Design review of the part shown in the three views and the two pictorial views. Dimensions are in mm from the part's minimum x, y and z. Coordinates: 2 decimals unless noted, no trailing zeros. Loops run counter-clockwise (first coordinate to the right, second up) from the corner with the lowest first, then second, coordinate; pieces in that order, holes last. Notation, with made-up numbers: (11.5, 31.25) - (15.5, 31.25) arc R21 ccw to (15.5, 47.25) - close; hole circle Ø6 at (16.5, -19.75). An arc over 180 degrees is marked (long way). One line per item, written item: value. Start each with the question number.
1. To check wall thickness, follow line 1 (Y direction, x = 25, z = 3.65); line 2 (Y direction, x = 15, z = 3.05); line 3 (Y direction, x = 2.25, z = 2.4). State the ranges of each line that lie inside material, in increasing order. Write a range as from..to.
2. Take a section at B-B, the plane z = 1.7. State the section outline as (x, y) points, and give its area (3 significant figures).
3. Insertion check: pin 1 (5 mm diameter, centred on x = 25, y = 112.5, fed in from +Z); pin 2 (1.5 mm diameter, centred on y = 123, z = 3.5, fed in from -X); pin 3 (2 mm diameter, centred on y = 26, z = 1.5, fed in from +X). Each pin has a flat end and moves straight along its axis. Give the tip position at first contact, or say it passes through.
4. Take a section at A-A, the plane x = 5. State the section outline as (y, z) points, and give its area (3 significant figures).
5. Take a section at C-C, the plane y = 12.5. State the section outline as (x, z) points.
6. Take a section at D-D, the plane x = 15. State the section outline as (y, z) points, and give its area (3 significant figures).
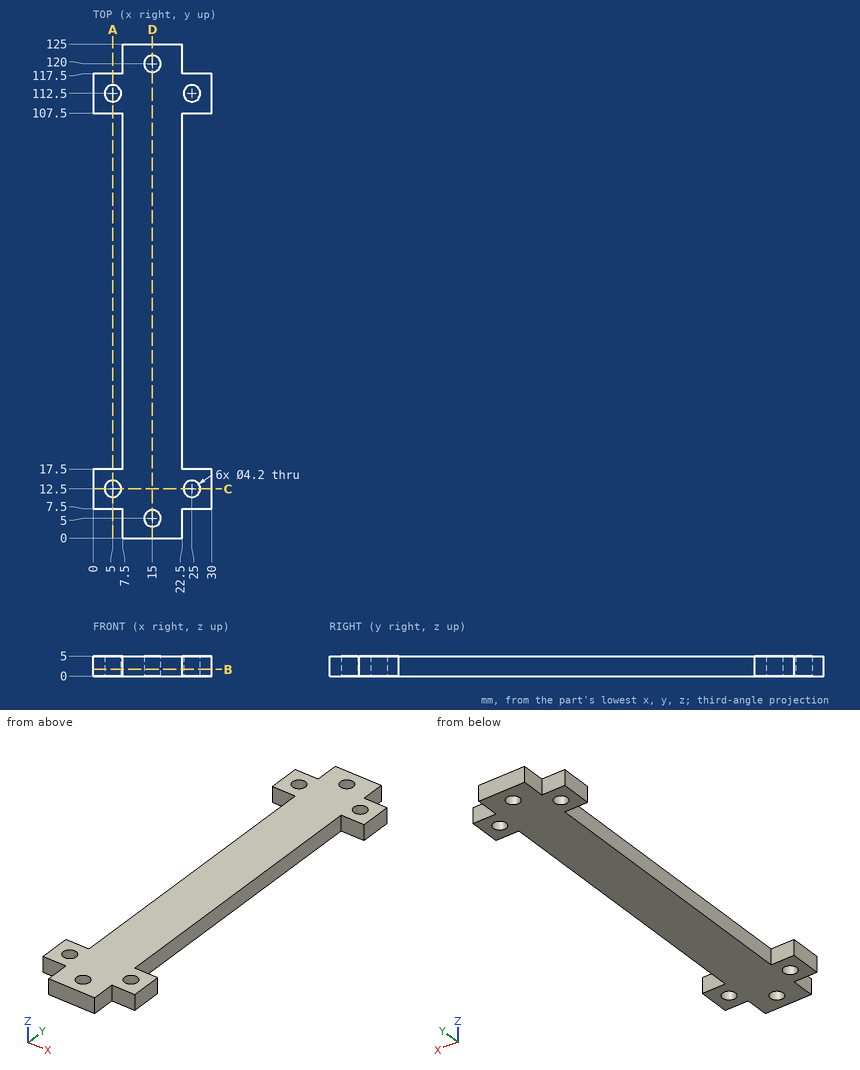
Solutions:
1. line 1: 7.5..10.4, 14.6..17.5, 107.5..110.4, 114.6..117.5
1. line 2: 0..2.9, 7.1..117.9, 122.1..125
1. line 3: 7.5..17.5, 107.5..117.5
2. outline: (0, 7.5) - (7.5, 7.5) - (7.5, 0) - (22.5, 0) - (22.5, 7.5) - (30, 7.5) - (30, 17.5) - (22.5, 17.5) - (22.5, 107.5) - (30, 107.5) - (30, 117.5) - (22.5, 117.5) - (22.5, 125) - (7.5, 125) - (7.5, 117.5) - (0, 117.5) - (0, 107.5) - (7.5, 107.5) - (7.5, 17.5) - (0, 17.5) - close; hole circle Ø4.2 at (5, 12.5); hole circle Ø4.2 at (5, 112.5); hole circle Ø4.2 at (15, 5); hole circle Ø4.2 at (15, 120); hole circle Ø4.2 at (25, 12.5); hole circle Ø4.2 at (25, 112.5)
2. area: 2,090 mm2
3. pin 1: z = 5
3. pin 2: x = 7.5
3. pin 3: x = 22.5
4. outline: (7.5, 0) - (10.4, 0) - (10.4, 5) - (7.5, 5) - close; (14.6, 0) - (17.5, 0) - (17.5, 5) - (14.6, 5) - close; (107.5, 0) - (110.4, 0) - (110.4, 5) - (107.5, 5) - close; (114.6, 0) - (117.5, 0) - (117.5, 5) - (114.6, 5) - close
4. area: 58.0 mm2
5. outline: (0, 0) - (2.9, 0) - (2.9, 5) - (0, 5) - close; (7.1, 0) - (22.9, 0) - (22.9, 5) - (7.1, 5) - close; (27.1, 0) - (30, 0) - (30, 5) - (27.1, 5) - close
6. outline: (0, 0) - (2.9, 0) - (2.9, 5) - (0, 5) - close; (7.1, 0) - (117.9, 0) - (117.9, 5) - (7.1, 5) - close; (122.1, 0) - (125, 0) - (125, 5) - (122.1, 5) - close
6. area: 583 mm2
